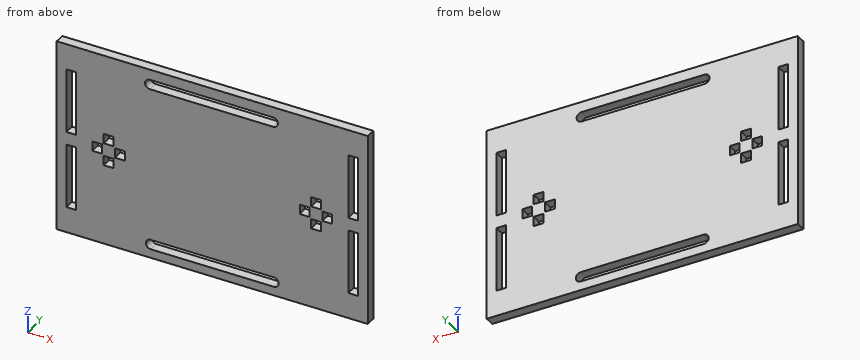
from build123d import *

# Parameters (mm, degrees)
SKETCH_1_W      = 3
SKETCH_1_H      = 20
SKETCH_1_H_2    = 3
EXTRUDE_2_DEPTH = 3


with BuildPart() as part:
    # 草图1 → 凸台-拉伸2 (new body)
    with BuildSketch(Plane(origin=(0, 0, 0), x_dir=(1, 0, 0), z_dir=(0, 1, 0))):
        Polygon((101.75, -0.25), (53.75, -0.25), (5.75, -0.25), (5.75, -60.25), (101.75, -60.25), align=None)
        with BuildLine():
            Line((34.5, -54), (53.75, -54))
            Line((53.75, -54), (72.5, -54))
            ThreePointArc((72.5, -54), (74, -55.5), (72.5, -57))
            Line((72.5, -57), (53.75, -57))
            Line((53.75, -57), (34.5, -57))
            ThreePointArc((34.5, -57), (33, -55.5), (34.5, -54))
        make_face(mode=Mode.SUBTRACT)
        with Locations((10.25, -42.25)):
            Rectangle(SKETCH_1_W, SKETCH_1_H, mode=Mode.SUBTRACT)
        with Locations((18.25, -30.25)):
            Rectangle(SKETCH_1_W, SKETCH_1_H_2, mode=Mode.SUBTRACT)
        with Locations((21.75, -33.75)):
            Rectangle(SKETCH_1_W, SKETCH_1_H_2, mode=Mode.SUBTRACT)
        with Locations((25.25, -30.25)):
            Rectangle(SKETCH_1_W, SKETCH_1_H_2, mode=Mode.SUBTRACT)
        with Locations((97.25, -42.25)):
            Rectangle(SKETCH_1_W, SKETCH_1_H, mode=Mode.SUBTRACT)
        with Locations((85.75, -33.75)):
            Rectangle(SKETCH_1_W, SKETCH_1_H_2, mode=Mode.SUBTRACT)
        with Locations((82.25, -30.25)):
            Rectangle(SKETCH_1_W, SKETCH_1_H_2, mode=Mode.SUBTRACT)
        with Locations((89.25, -30.25)):
            Rectangle(SKETCH_1_W, SKETCH_1_H_2, mode=Mode.SUBTRACT)
        with Locations((21.75, -26.75)):
            Rectangle(SKETCH_1_W, SKETCH_1_H_2, mode=Mode.SUBTRACT)
        with Locations((10.25, -18.25)):
            Rectangle(SKETCH_1_W, SKETCH_1_H, mode=Mode.SUBTRACT)
        with Locations((85.75, -26.75)):
            Rectangle(SKETCH_1_W, SKETCH_1_H_2, mode=Mode.SUBTRACT)
        with Locations((97.25, -18.25)):
            Rectangle(SKETCH_1_W, SKETCH_1_H, mode=Mode.SUBTRACT)
        with BuildLine():
            Line((34.75, -3), (53.75, -3))
            Line((53.75, -3), (72.75, -3))
            ThreePointArc((72.75, -3), (74.25, -4.5), (72.75, -6))
            Line((72.75, -6), (53.75, -6))
            Line((53.75, -6), (34.75, -6))
            ThreePointArc((34.75, -6), (33.25, -4.5), (34.75, -3))
        make_face(mode=Mode.SUBTRACT)
    extrude(amount=EXTRUDE_2_DEPTH)


solid = part.part
Can you work these out from the model? Positions are in its coordinate system, mm. Coordinates: 2 decimals unless noted, no trailing zeros. Write each loop counter-clockwise with the first axis right and the second up, starting at its lowest first coordinate (ties: lowest second). Pieces come first, ordered by that corner, then holes.
Q1. Imagine slicing it at B-B, the plane z = 55.5. List the corners of the cut face in (x, y) for me, plus the area to 3 significant figures.
Results found:
outline: (5.75, 0) - (33, 0) - (33, 3) - (5.75, 3) - close; (74, 0) - (101.75, 0) - (101.75, 3) - (74, 3) - close
area: 165 mm2
Q2. Please list where these lines run through material, in increasing order: L1, parallel to Z at x = 62.5, y = 0.15; L2, parallel to X at y = 1.2, z = 43; L3, parallel to X at y = 1.05, z = 26.
Results found:
L1: z = 0.25 to 3, 6 to 54, 57 to 60.25
L2: x = 5.75 to 8.75, 11.75 to 95.75, 98.75 to 101.75
L3: x = 5.75 to 8.75, 11.75 to 20.25, 23.25 to 84.25, 87.25 to 95.75, 98.75 to 101.75
Q3. Imagine slicing it at A-A, the plane z = 47. List the corners of the cut face in (x, y) for me.
Results found:
outline: (5.75, 0) - (8.75, 0) - (8.75, 3) - (5.75, 3) - close; (11.75, 0) - (95.75, 0) - (95.75, 3) - (11.75, 3) - close; (98.75, 0) - (101.75, 0) - (101.75, 3) - (98.75, 3) - close
Q4. Imagine slicing it at C-C, the plane y = 2. Count the separate pieces of the cut face and the enclosed holes in it, plus the area to 3 significant figures.
Results found:
separate pieces: 1
enclosed holes: 14
area: 5,210 mm2
Q5. For P1, Ø4, axis at x = 41.5, z = 36.5, coming from the -Y side, with a flat end and sliding along its axis, tell me the tip position at first contact or that it passes through.
Results found:
P1: stops at y = 0
